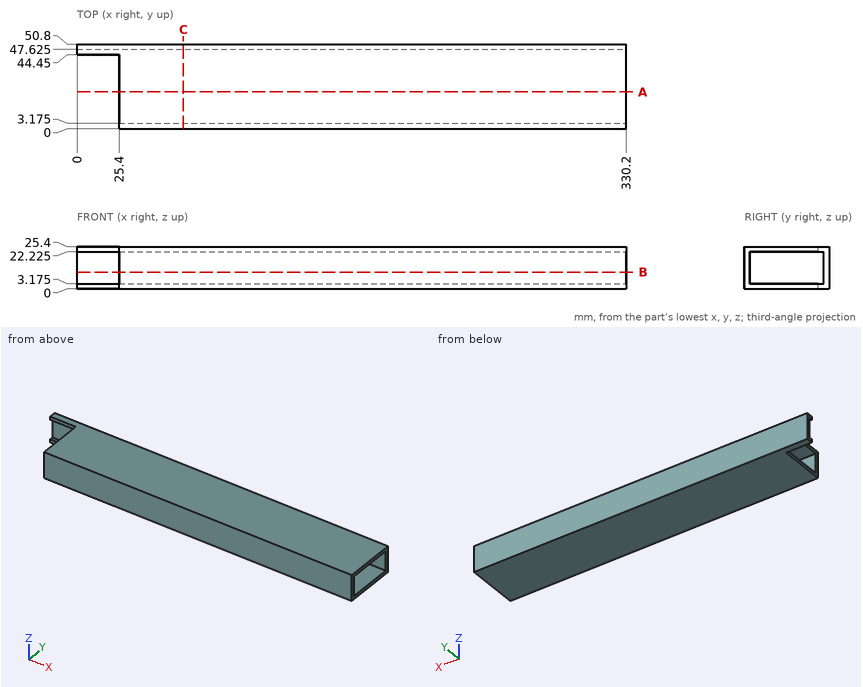
Design review of the part shown in the three views and the two pictorial views. Dimensions are in mm from the part's minimum x, y and z. Give positions to 0.01 mm unless a question says otherwise; leave off trailing zeros. Order: outer loops, then holes, each group sorted by start corner. A loop starts at its lowest first (then second) coordinate and runs counter-clockwise, first axis right, second up. Notation, with made-up numbers: M 79,-34 L 107,-34 A18 cw 107,-5 Z; hole C 6,-1 d1. An arc over 180 degrees is marked long. Answer in a Markdown table with one row per item. Add a question column.
(1) Consider section B-B on z = 10. State the section outline as (x, y) points (3 decimals).
(2) Consider section C-C on x = 64. State the section outline as (y, z) points (3 decimals), and give its area (3 significant figures).
(3) For pin 1 (2 mm diameter, centred on x = 217, z = 5, fed in from -Y); pin 2 (6 mm diameter, centred on y = 42, z = 17, fed in from -X); pin 3 (1 mm diameter, centred on x = 18.5, z = 1.5, fed in from -Y), all flat-tipped, find the tip position at first contact; note any pin that passes through.
(4) Consider section A-A on y = 22. State the section outline as (x, z) points (3 decimals), and give its area (3 significant figures).
(5) Wall thickness on probe 1 along Y at (x, z) = (82, 9.25) (3 decimals); probe 2 along Z at (x, y) = (184, 42) (3 decimals); probe 3 along X at (y, z) = (39, 2.75): over which ranges is each line inside the solid? List them lowest first. Write a range as [from, to].
Evaluation:
| question | item | result |
|---|---|---|
| 1 | outline | M 0,47.625 L 330.2,47.625 L 330.2,50.8 L 0,50.8 Z; M 25.4,0 L 330.2,0 L 330.2,3.175 L 25.4,3.175 Z |
| 2 | outline | M 0,0 L 50.8,0 L 50.8,25.4 L 0,25.4 Z; hole M 3.175,3.175 L 47.625,3.175 L 47.625,22.225 L 3.175,22.225 Z |
| 2 | area | 444 mm^2 |
| 3 | pin 1 | stops at y = 0 |
| 3 | pin 2 | passes through |
| 3 | pin 3 | stops at y = 44.45 |
| 4 | outline | M 25.4,0 L 330.2,0 L 330.2,3.175 L 25.4,3.175 Z; M 25.4,22.225 L 330.2,22.225 L 330.2,25.4 L 25.4,25.4 Z |
| 4 | area | 1,940 mm^2 |
| 5 | probe 1 | y = [0, 3.175], [47.625, 50.8] |
| 5 | probe 2 | z = [0, 3.175], [22.225, 25.4] |
| 5 | probe 3 | x = [25.4, 330.2] |
